```python
from build123d import *

# Parameters (mm, degrees)
F0_W          = 24
F0_H          = 14
F1_DEPTH      = 2.4
F3_R          = 6
F4_DEPTH      = 8
F5_R          = 6
F6_DEPTH      = 4
F2_R          = 2
F7_DEPTH      = 2.401
F7_DEPTH_BACK = 8.001
F8_R          = 2
F9_DEPTH      = 6.401
F10_R         = 3.5
F11_DEPTH     = 2
F12_R         = 4
F13_DEPTH     = 2
F14_T1_DEPTH  = 37.4
F15_R         = 6


# Not quite as in the source:
# - a fillet or chamfer that OpenCascade refuses, or shapes differently, is made with other operations: its cross-section is extruded or revolved along the edge and cut away or added


with BuildPart() as f1:
    # F0 (on Top) → F1 (new body)
    with BuildSketch(Plane.XY):
        with Locations((-3.2606057666, 7)):
            Rectangle(F0_W, F0_H)
    extrude(amount=F1_DEPTH)

    # F3 (on face) → F4 (join)
    with BuildSketch(Plane.XY.offset(2.4)):
        with Locations((-9.2606057666, 7)):
            Circle(F3_R)
    extrude(amount=F4_DEPTH)

    # F5 (on face) → F6 (join)
    with BuildSketch(Plane.XY.offset(2.4)):
        with Locations((1.7393942334, 7)):
            Circle(F5_R)
    extrude(amount=F6_DEPTH)

    # F2 (on face) → F7 (cut, two sides)
    with BuildSketch(Plane.XY.offset(2.4)) as f7_sk:
        with Locations((-9.2606057666, 7)):
            Circle(F2_R)
    extrude(amount=-F7_DEPTH, mode=Mode.SUBTRACT)
    extrude(f7_sk.sketch, amount=F7_DEPTH_BACK, mode=Mode.SUBTRACT)

    # F8 (on face) → F9 (cut, through all)
    with BuildSketch(Plane.XY.offset(6.4)):
        with Locations((1.7393942334, 7)):
            Circle(F8_R)
    extrude(amount=-F9_DEPTH, mode=Mode.SUBTRACT)

    # F10 (on face) → F11 (cut)
    with BuildSketch(Plane(origin=(0, 0, 0), x_dir=(1, 0, 0), z_dir=(0, 0, -1))):
        with Locations((1.7393942334, -7)):
            Circle(F10_R)
    extrude(amount=-F11_DEPTH, mode=Mode.SUBTRACT)

    # F12 (on face) → F13 (cut)
    with BuildSketch(Plane.XY.offset(6.4)):
        with Locations((1.7393942334, 7)):
            Circle(F12_R)
    extrude(amount=-F13_DEPTH, mode=Mode.SUBTRACT)

    # F14: fillet of radius 7 on 4 edges, made by hand

    # F14_s2 → F14_t1 (cut)
    with BuildSketch(Plane.XY.offset(-17.5)):
        with BuildLine():
            ThreePointArc((-8.2606057666, 14), (-13.2103532349, 11.9497474683), (-15.2606057666, 7))
            Line((-15.2606057666, 7), (-15.2606057666, 14))
            Line((-15.2606057666, 14), (-8.2606057666, 14))
        make_face()
        with BuildLine():
            ThreePointArc((-15.2606057666, 7), (-13.2103532349, 2.0502525317), (-8.2606057666, 0))
            Line((-8.2606057666, 0), (-15.2606057666, 0))
            Line((-15.2606057666, 0), (-15.2606057666, 7))
        make_face()
        with BuildLine():
            ThreePointArc((8.7393942334, 7), (6.6891417017, 2.0502525317), (1.7393942334, 0))
            Line((1.7393942334, 0), (8.7393942334, 0))
            Line((8.7393942334, 0), (8.7393942334, 7))
        make_face()
        with BuildLine():
            ThreePointArc((1.7393942334, 14), (6.6891417017, 11.9497474683), (8.7393942334, 7))
            Line((8.7393942334, 7), (8.7393942334, 14))
            Line((8.7393942334, 14), (1.7393942334, 14))
        make_face()
    extrude(amount=F14_T1_DEPTH, mode=Mode.SUBTRACT)

    # F15
    f15_edges = [f1.edges().sort_by_distance(p)[0] for p in [
        (-3.760606, 4.602084, 4.4),
        (-3.760606, 9.397916, 4.4),
    ]]
    fillet(f15_edges, radius=F15_R)


solid = f1.part
```
Geometry check sheet. Reference: the model listing, model coordinates, mm. A direction names the side the tool comes from. Coordinates: 2 decimals unless noted, no trailing zeros. Order: outer loops, then holes, each group sorted by start corner. A loop starts at its lowest first (then second) coordinate and runs counter-clockwise, first axis right, second up.
Q1. Draft check along Y on faces 1 (the face through (3, 9, 4.4)), 2 (the face through (1.479, 8.983, 3.217)), 3 (the face through (7.737, 6.828, 4.372)), 4 (the face through (-3, 7, 6.4)). Enter one of: released by +Y, released by -Y, zero draft, split by the parting line, or undercut.
Reply:
face 1: undercut
face 2: undercut
face 3: split by the parting line
face 4: zero draft
Q2. Depth check by flat-ended pin: pin 1 Ø1.5 at (y, z) = (10, 8) entering from +X; pin 2 Ø6 at (x, z) = (-10.5, 9) entering from +Y; pin 3 Ø4.5 at (x, y) = (1.74, 7) entering from +Z. Enter the tip coordinate at first touch or a pass-through.
Reply:
pin 1: stops at x = -3.7
pin 2: stops at y = 13
pin 3: stops at z = 4.4
Q3. Sectioned sample at C-C on y = 5.75. Give the number of separate pieces and of enclosed holes in the cut face, and give its area (3 significant figures).
Reply:
separate pieces: 3
enclosed holes: 0
area: 127 mm2
Q4. Sectioned sample at B-B on x = 3.5. Record the cut outline in (y, z), and give its area (3 significant figures).
Reply:
outline: (0.23, 0) - (3.98, 0) - (3.98, 2) - (6.05, 2) - (6.05, 4.4) - (3.41, 4.4) - (3.41, 6.4) - (1.26, 6.4) - (1.26, 2.4) - (0.23, 2.4) - close; (7.95, 2) - (10.02, 2) - (10.02, 0) - (13.77, 0) - (13.77, 2.4) - (12.74, 2.4) - (12.74, 6.4) - (10.59, 6.4) - (10.59, 4.4) - (7.95, 4.4) - close
area: 47.4 mm2
Q5. Sectioned sample at D-D on z = 7.75. Record the cut outline in (x, y).
Reply:
outline: circle Ø12 at (-9.26, 7); hole circle Ø4 at (-9.26, 7)
Q6. Tool access check on faces 5 (the face through (-2.4, 1.8, 2.4)), 6 (the face through (3, 9, 2)), 7 (the face through (-7, 7, 10.4)). Record the directions out of +Z, -Z, +X, -X, +Y, -Y that give a thin tool (end or side, any length) a straight path to the whole face; none if there is none.
Reply:
face 5: +Z
face 6: -Z
face 7: +Z, +X, -X, +Y, -Y
Q7. Thickness scan on probe 1 along X at (y, z) = (7, 0.6); probe 2 along X at (y, z) = (6.75, 0.5); probe 3 along Z at (x, y) = (0, 8.5). Record the ranges inside material, lowest first.
Reply:
probe 1: x = -15.26 to -11.26, -7.26 to -1.76, 5.24 to 8.74
probe 2: x = -15.26 to -11.24, -7.28 to -1.75, 5.23 to 8.73
probe 3: z = 2 to 4.4
Q8. Sectioned sample at A-A on z = 1.5. Record the cut outline in (x, y), and give its area (3 significant figures).
Reply:
outline: (-8.26, 0) - (1.74, 0) arc R7 ccw to (1.74, 14) - (-8.26, 14) arc R7 ccw to start; hole circle Ø4 at (-9.26, 7); hole circle Ø7 at (1.74, 7)
area: 243 mm2
